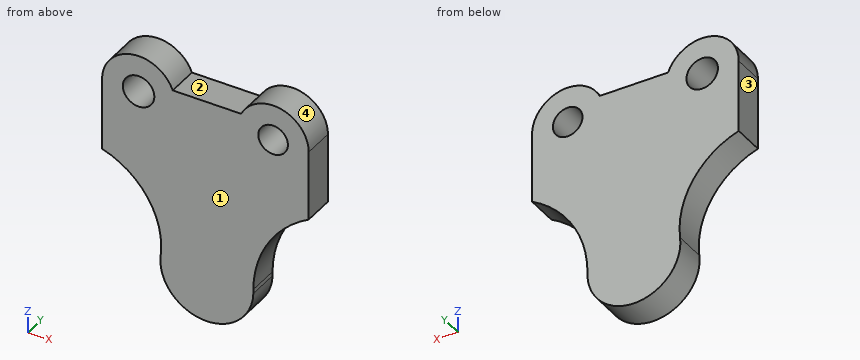
from build123d import *

# Parameters (mm, degrees)
F0_R     = 12.639572
F0_R_2   = 11.88315
F1_DEPTH = 25.4


with BuildPart() as f1:
    # F0 (on Front) → F1 (new body)
    with BuildSketch(Plane.XZ):
        with BuildLine():
            Line((27.448043, 68.576015), (-27.390932, 68.576015))
            ThreePointArc((-27.390932, 68.576015), (-60.105703, 86.910739), (-84.08658, 58.077842))
            Line((-84.08658, 58.077842), (-84.08658, 0))
            ThreePointArc((-84.08658, 0), (-47.588606, -27.462088), (-37.051876, -71.905824))
            ThreePointArc((-37.051876, -71.905824), (-2.635407, -113.336224), (37.278298, -77.171771))
            ThreePointArc((37.278298, -77.171771), (37.23573, -75.532835), (37.225122, -73.893381))
            ThreePointArc((37.225122, -73.893381), (49.262547, -30.813467), (81.686439, 0))
            Line((81.686439, 0), (81.680074, 56.022676))
            ThreePointArc((81.680074, 56.022676), (59.553216, 83.853143), (27.448043, 68.576015))
        make_face()
        with Locations((-54.767519, 58.081741)):
            Circle(F0_R, mode=Mode.SUBTRACT)
        with Locations((53.110417, 56.019429)):
            Circle(F0_R_2, mode=Mode.SUBTRACT)
    extrude(amount=F1_DEPTH)


solid = f1.part
For this review, take the finished solid that the model builds, in its own axes (mm). Face numbers are marked on the shaded views. Round coordinates to 2 decimals unless told otherwise and drop trailing zeros. Loops run counter-clockwise (first coordinate to the right, second up) from the corner with the lowest first, then second, coordinate; pieces in that order, holes last. Notation, with made-up numbers: (-39.75, 60) - (-3.75, 60) arc R16 cw to (-3.75, 91) - close; hole circle Ø8 at (64, -17.5). An arc over 180 degrees is marked (long way). Use one line per item in the form item = value.
Item 1: Consider section B-B on y = -22.25. Write out the cut boundary in (x, z).
Answers:
outline = (-84.09, 0) arc R67.25 cw to (-37.05, -71.91) arc R37.29 ccw (long way) to (37.28, -77.17) arc R84.09 cw to (37.23, -73.89) arc R84.09 cw to (81.69, 0) - (81.68, 56.02) arc R28.57 ccw to (27.45, 68.58) - (-27.39, 68.58) arc R29.32 ccw to (-84.09, 58.08) - close; hole circle Ø25.28 at (-54.77, 58.08); hole circle Ø23.77 at (53.11, 56.02)
Item 2: For line 1 (X direction, y = -9.5, z = 56.5); line 2 (X direction, y = -14.5, z = 41); line 3 (Z direction, x = -66, y = -2), list the stretches that pass through material, from the lowest coordinate up.
Answers:
line_1 = -84.09 to -67.31, -42.23 to 41.24, 64.98 to 81.68
line_2 = -84.09 to 81.68
line_3 = -8.7 to 52.29, 63.88 to 85.16
Item 3: Clearance check with flat-ended pins moving along their axes: P1, Ø14.5, axis at x = 53.11, z = 56.02, coming from the +Y side; P2, Ø2, axis at y = -3.5, z = -44.5, coming from the +X side; P3, Ø10, axis at x = 37.5, y = -8.5, coming from the -Z side; P4, Ø10, axis at x = -5.5, y = -9, coming from the +Z side. State where each tip first meets the part, or that it passes through.
Answers:
P1 = through
P2 = 43.02
P3 = -94.43
P4 = 68.58
Item 4: Consider section D-D on z = -8. Write out the cut boundary in (x, y), then the cut area to 3 significant figures.
Answers:
outline = (-67.05, -25.4) - (69.42, -25.4) - (69.42, 0) - (-67.05, 0) - close
area = 3,470 mm^2
Item 5: Mouldability with a two-part tool opening along X and no side actions: class the marked faces 1, 2, 3 and 4 as +X half, -X half, draft (parallel to the pull), parting line (faces both ways), or undercut.
Answers:
face_1 = draft
face_2 = undercut
face_3 = -X half
face_4 = undercut
Item 6: Consider section A-A on x = -60. Write out the cut boundary in (y, z).
Answers:
outline = (-25.4, -13.3) - (0, -13.3) - (0, 46.58) - (-25.4, 46.58) - close; (-25.4, 69.59) - (0, 69.59) - (0, 86.93) - (-25.4, 86.93) - close
Item 7: Consider section C-C on x = 44.5. Write out the cut boundary in (y, z).
Answers:
outline = (-25.4, -39.95) - (0, -39.95) - (0, 47.83) - (-25.4, 47.83) - close; (-25.4, 64.21) - (0, 64.21) - (0, 83.26) - (-25.4, 83.26) - close
